Verification items for the finished model (mm, model axes). Coordinates: 2 decimals unless noted, no trailing zeros. Write each loop counter-clockwise with the first axis right and the second up, starting at its lowest first coordinate (ties: lowest second). Pieces come first, ordered by that corner, then holes. Notation, with made-up numbers: M 3.25,55 L 44.25,55 A20 ccw 44.25,75 Z; hole C 86.5,10 d9. An arc over 180 degrees is marked long. Answer in a Markdown table with one row per item.
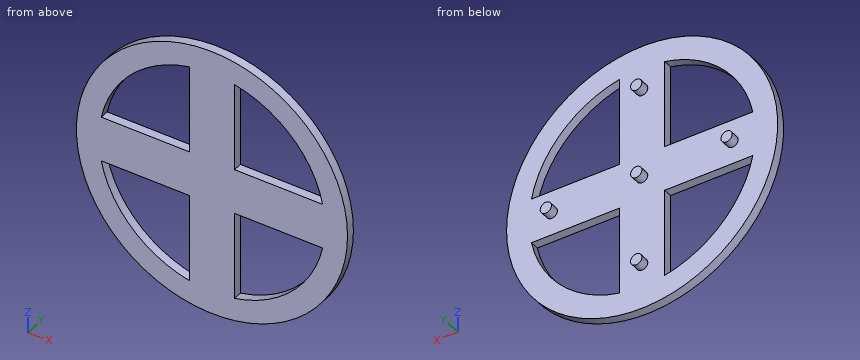
from build123d import *

# Parameters (mm, degrees)
SKETCH1_R           = 38.1
BOSS_EXTRUDE1_DEPTH = 2.5
SKETCH2_R           = 1.5875
BOSS_EXTRUDE2_DEPTH = 2.5


with BuildPart() as part:
    # Sketch1 → Boss-Extrude1 (new body)
    with BuildSketch(Plane(origin=(0, 0, 0), x_dir=(1, 0, 0), z_dir=(0, 1, 0))):
        Circle(SKETCH1_R)
        with BuildLine():
            ThreePointArc((6.35, -31.108519733), (22.450640303, -22.450640303), (31.108519733, -6.35))
            Line((31.108519733, -6.35), (6.35, -6.35))
            Line((6.35, -6.35), (6.35, -31.108519733))
        make_face(mode=Mode.SUBTRACT)
        with BuildLine():
            ThreePointArc((-31.108519733, -6.35), (-22.450640303, -22.450640303), (-6.35, -31.108519733))
            Line((-6.35, -31.108519733), (-6.35, -6.35))
            Line((-6.35, -6.35), (-31.108519733, -6.35))
        make_face(mode=Mode.SUBTRACT)
        with BuildLine():
            ThreePointArc((-6.35, 31.108519733), (-22.450640303, 22.450640303), (-31.108519733, 6.35))
            Line((-31.108519733, 6.35), (-6.35, 6.35))
            Line((-6.35, 6.35), (-6.35, 31.108519733))
        make_face(mode=Mode.SUBTRACT)
        with BuildLine():
            ThreePointArc((31.108519733, 6.35), (22.450640303, 22.450640303), (6.35, 31.108519733))
            Line((6.35, 31.108519733), (6.35, 6.35))
            Line((6.35, 6.35), (31.108519733, 6.35))
        make_face(mode=Mode.SUBTRACT)
    extrude(amount=BOSS_EXTRUDE1_DEPTH)

    # Sketch2 → Boss-Extrude2 (add)
    with BuildSketch(Plane(origin=(0, 2.5, 0), x_dir=(1, 0, 0), z_dir=(0, 1, 0))):
        Circle(SKETCH2_R)
        with Locations((-25.4, 0)):
            Circle(SKETCH2_R)
        with Locations((0, 25.4)):
            Circle(SKETCH2_R)
        with Locations((25.4, 0)):
            Circle(SKETCH2_R)
        with Locations((0, -25.4)):
            Circle(SKETCH2_R)
    extrude(amount=BOSS_EXTRUDE2_DEPTH)


solid = part.part
1) Thickness scan on L1, parallel to Z at x = 0, y = 4.2; L2, parallel to X at y = 1.15, z = -26; L3, parallel to X at y = 2.4, z = -12.5. Record the ranges inside material, lowest first. Write a range as [from, to].
Response values:
| item | result |
|---|---|
| L1 | z = [-26.99, -23.81], [-1.59, 1.59], [23.81, 26.99] |
| L2 | x = [-27.85, -18.22], [-6.35, 6.35], [18.22, 27.85] |
| L3 | x = [-35.99, -29.19], [-6.35, 6.35], [29.19, 35.99] |
2) Sectioned sample at A-A (y = 0.85). Record the cut outline in (x, z), then the cut area to 3 significant figures.
Response values:
| item | result |
|---|---|
| outline | C 0,0 d76.2; hole M -31.11,-6.35 A31.75 ccw -6.35,-31.11 L -6.35,-6.35 Z; hole M -31.11,6.35 L -6.35,6.35 L -6.35,31.11 A31.75 ccw Z; hole M 6.35,-31.11 A31.75 ccw 31.11,-6.35 L 6.35,-6.35 Z; hole M 6.35,6.35 L 31.11,6.35 A31.75 ccw 6.35,31.11 Z |
| area | 2,830 mm² |
3) Sectioned sample at B-B (x = 25.4). Record the cut outline in (y, z).
Response values:
| item | result |
|---|---|
| outline | M 0,-28.4 L 2.5,-28.4 L 2.5,-19.05 L 0,-19.05 Z; M 0,-6.35 L 2.5,-6.35 L 2.5,-1.59 L 5,-1.59 L 5,1.59 L 2.5,1.59 L 2.5,6.35 L 0,6.35 Z; M 0,19.05 L 2.5,19.05 L 2.5,28.4 L 0,28.4 Z |
4) Depth check by flat-ended pin: pin 1 (3 mm diameter, centred on x = -14, y = 1, fed in from -Z); pin 2 (10 mm diameter, centred on x = -7.5, z = -8, fed in from -Y); pin 3 (3 mm diameter, centred on x = 17.5, y = 1.5, fed in from -Z); pin 4 (1.5 mm diameter, centred on x = -11.5, z = 29.5, fed in from +Y). Enter the tip coordinate at first touch or a pass-through.
Response values:
| item | result |
|---|---|
| pin 1 | stops at z = -35.99 |
| pin 2 | stops at y = 0 |
| pin 3 | stops at z = -34.58 |
| pin 4 | stops at y = 2.5 |
5) Sectioned sample at D-D (x = 0). Record the cut outline in (y, z), then the cut area to 3 significant figures.
Response values:
| item | result |
|---|---|
| outline | M 0,-38.1 L 2.5,-38.1 L 2.5,-26.99 L 5,-26.99 L 5,-23.81 L 2.5,-23.81 L 2.5,-1.59 L 5,-1.59 L 5,1.59 L 2.5,1.59 L 2.5,23.81 L 5,23.81 L 5,26.99 L 2.5,26.99 L 2.5,38.1 L 0,38.1 Z |
| area | 214 mm² |
6) Sectioned sample at C-C (z = 11). Record the cut outline in (x, y), then the cut area to 3 significant figures.
Response values:
| item | result |
|---|---|
| outline | M -36.48,0 L -29.78,0 L -29.78,2.5 L -36.48,2.5 Z; M -6.35,0 L 6.35,0 L 6.35,2.5 L -6.35,2.5 Z; M 29.78,0 L 36.48,0 L 36.48,2.5 L 29.78,2.5 Z |
| area | 65.2 mm² |
